Input: part model. Units: mm. Frame: model coordinates. A direction names the side the tool comes from. Coordinates: 2 decimals unless noted, no trailing zeros. Order: outer loops, then holes, each group sorted by start corner. A loop starts at its lowest first (then second) coordinate and runs counter-clockwise, first axis right, second up.
from build123d import *

# Parameters (mm, degrees)
EXTRUDE_2_DEPTH          = 10
CUT_EXTRUDE_1_DEPTH      = 55.083263276
CUT_EXTRUDE_1_DEPTH_BACK = 55.083263276
SKETCH_2_R               = 2
EXTRUDE_4_DEPTH          = 20
SKETCH_4_R               = 2.5
CUT_EXTRUDE_2_DEPTH      = 20
FILLET_1_R               = 1


with BuildPart() as part:
    # Sketch 1 → Extrude 2 (new body)
    with BuildSketch(Plane(origin=(0, 0, 0), x_dir=(1, 0, 0), z_dir=(0, 1, 0))):
        with BuildLine():
            Line((19.976699203, -29.999990951), (17.304982924, -29.999990951))
            Line((17.304982924, -29.999990951), (31.312388487, -5.781912211))
            ThreePointArc((31.312388487, -5.781912211), (33.145618934, -3.952237958), (35.648339397, -3.28528067))
            Line((35.648339397, -3.28528067), (38.994935663, -3.290479232))
            ThreePointArc((38.994935663, -3.290479232), (39.702496567, -2.998684777), (39.996487843, -2.292033825))
            Line((39.996487843, -2.292033825), (39.999773177, -0.177085839))
            ThreePointArc((39.999773177, -0.177085839), (39.707978722, 0.530475065), (39.00132777, 0.82446634))
            Line((39.00132777, 0.82446634), (34.146000565, 0.832008547))
            Line((34.146000565, 0.832008547), (26.001089345, 0.844660753))
            ThreePointArc((26.001089345, 0.844660753), (25.295095717, 0.554425262), (24.999553807, -0.1493635))
            ThreePointArc((24.999553807, -0.1493635), (-0.019417331, -24.999992459), (-24.999755664, -0.110529363))
            ThreePointArc((-24.999755664, -0.110529363), (-25.294203962, 0.593717641), (-25.999745891, 0.885049463))
            Line((-25.999745891, 0.885049463), (-39, 0.885049463))
            ThreePointArc((-39, 0.885049463), (-39.707106781, 0.592156244), (-40, -0.114950537))
            Line((-40, -0.114950537), (-40, -2.229901074))
            ThreePointArc((-40, -2.229901074), (-39.707106781, -2.937007856), (-39, -3.229901074))
            Line((-39, -3.229901074), (-35.653399696, -3.229901074))
            ThreePointArc((-35.653399696, -3.229901074), (-33.151718295, -3.900745249), (-31.32133225, -5.733265009))
            Line((-31.32133225, -5.733265009), (-17.343803649, -29.98653823))
            Line((-17.343803649, -29.98653823), (-20.023300797, -29.999990951))
            Line((-20.023300797, -29.999990951), (-20.023300797, -34.999990951))
            Line((-20.023300797, -34.999990951), (19.976699203, -34.999990951))
            Line((19.976699203, -34.999990951), (19.976699203, -29.999990951))
        make_face()
    extrude(amount=EXTRUDE_2_DEPTH)

    # Sketch 2 → Cut-Extrude 1 (cut, two sides: drawn at the far end of the back side and taken through both)
    with BuildSketch(Plane.XY.offset(-CUT_EXTRUDE_1_DEPTH_BACK)):
        with Locations(Location((-35, 5, 0), (0, 0, 250.931408375))):
            Circle(SKETCH_2_R)
        with Locations(Location((35, 5, 0), (0, 0, 180))):
            Circle(SKETCH_2_R)
    extrude(amount=CUT_EXTRUDE_1_DEPTH + CUT_EXTRUDE_1_DEPTH_BACK, mode=Mode.SUBTRACT)

    # Sketch 1_6 → Extrude 4 (add)
    with BuildSketch(Plane(origin=(0, 0, 0), x_dir=(1, 0, 0), z_dir=(0, 1, 0))):
        Polygon((17.304982924, -29.999990951), (17.297202054, -30.013443673), (-0.023300797, -29.999990951), (-17.343803649, -29.98653823), (-20.023300797, -29.999990951), (-20.023300797, -34.999990951), (19.976699203, -34.999990951), (19.976699203, -29.999990951), align=None)
    extrude(amount=EXTRUDE_4_DEPTH)

    # Sketch 4 → Cut-Extrude 2 (cut)
    with BuildSketch(Plane.XY.offset(34.999990951)):
        with Locations((-10, 16)):
            Circle(SKETCH_4_R)
        with Locations((10, 16)):
            Circle(SKETCH_4_R)
    extrude(amount=-CUT_EXTRUDE_2_DEPTH, mode=Mode.SUBTRACT)

    # Fillet 1
    fillet_1_edges = [part.edges().sort_by_distance(p)[0] for p in [
        (18.640841063, 0, 29.999990951),
        (19.976699203, 0, 32.499990951),
        (-0.023300797, 0, 34.999990951),
        (-20.023300797, 0, 32.499990951),
        (-18.683552223, 0, 29.99326459),
        (19.976699203, 10, 29.999990951),
        (19.976699203, 10, 34.999990951),
        (-20.023300797, 10, 34.999990951),
        (-20.023300797, 10, 29.999990951),
        (-20.023300797, 20, 32.499990951),
        (-0.023300797, 20, 34.999990951),
        (19.976699203, 20, 32.499990951),
        (18.640841063, 20, 29.999990951),
        (17.301092489, 20, 30.006717312),
        (-0.023300797, 20, 29.999990951),
        (-18.683552223, 20, 29.99326459),
    ]]
    fillet(fillet_1_edges, radius=FILLET_1_R)


solid = part.part
Item 1: Cut plane C-C on x = -34. Return loops of the section in (y, z).
Response values:
outline: (0, -0.89) - (3.27, -0.89) - (3.27, 3.51) - (0, 3.51) - close; (6.73, -0.89) - (10, -0.89) - (10, 3.51) - (6.73, 3.51) - close
Item 2: Cut plane B-B on y = 4. Count the separate pieces of the cut face and the enclosed holes in it, then the cut area to 3 significant figures.
Response values:
separate pieces: 3
enclosed holes: 0
area: 815 mm2
Item 3: Ray query, probe 1 along X at (y, z) = (5, 0.7); probe 2 along X at (y, z) = (16, 31.3); probe 3 along Y at (x, z) = (10, 31). Return the intervals inside material, ascending.
Response values:
probe 1: x = -40 to -37, -33 to -24.99, 24.99 to 33, 37 to 40
probe 2: x = -20.02 to -12.5, -7.5 to 7.5, 12.5 to 19.98
probe 3: y = 0 to 13.5, 18.5 to 20
Item 4: Cut plane A-A on z = 11. Return loops of the section in (x, y), then the cut area to 3 significant figures.
Response values:
outline: (-28.29, 0) - (-22.45, 0) - (-22.45, 10) - (-28.29, 10) - close; (22.45, 0) - (28.29, 0) - (28.29, 10) - (22.45, 10) - close
area: 117 mm2
Item 5: Draft query along Y for faces 4 (the face through (23.9, 4.9, 18.6)), 5 (the face through (0, 10, 26)), 6 (the face through (-33.24, 5.95, 1.52)). Return one class per face: pulls with the +Y half, pulls with the -Y half, needs draft (parallel to the pull), parting line crosses it, or undercut.
Response values:
face 4: needs draft
face 5: pulls with the +Y half
face 6: undercut
Item 6: Pin query (flat end, axial travel): pin 1 Ø1.5 at (y, z) = (10, 32) entering from -X; pin 2 Ø8 at (y, z) = (15.5, 4) entering from +X; pin 3 Ø6 at (x, y) = (-10, 16) entering from -Z; pin 4 Ø5 at (x, y) = (-18, 9) entering from -Z. Return the tip coordinate at first contact, or that it passes through.
Response values:
pin 1: stops at x = -20.02
pin 2: passes through
pin 3: stops at z = 29.99
pin 4: stops at z = 14.31
Item 7: Access query for faces 1 (the face through (19.977, 10, 33)), 2 (the face through (-37.4, 4.9, 3.23)), 3 (the face through (33.153, 5.766, 1.569)). Directions: +Z, -Z, +X, -X, +Y, -Y. A direction counts if a zero-diameter tool reaches every point of the face in a straight line with its end or side. Return the directions, or none.
Response values:
face 1: +Z, +X, +Y, -Y
face 2: +Z, -X, +Y, -Y
face 3: +Z, -Z
